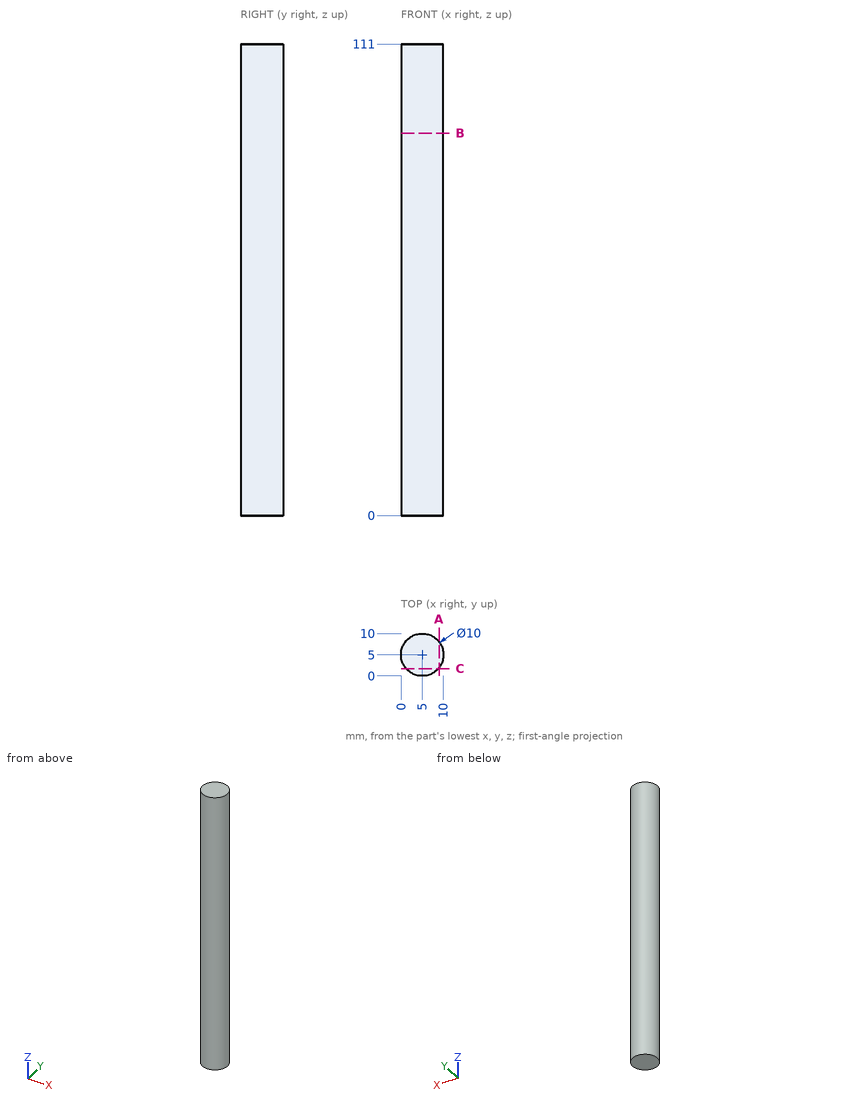
Print and shaded views of the part. All mm, measured from the part's lowest x, y and z. Round coordinates to 2 decimals unless told otherwise and drop trailing zeros. Write each loop counter-clockwise with the first axis right and the second up, starting at its lowest first coordinate (ties: lowest second). Pieces come first, ordered by that corner, then holes. Notation, with made-up numbers: (-16.5, 42) - (40.5, 42) arc R21 ccw to (40.5, 57) - close; hole circle Ø10 at (66, -32). An arc over 180 degrees is marked (long way). Use CSV: the item, a comma, the result in double quotes. Start each with the question number.
Item 1: Pin check, flat tips, straight feed: P1, Ø6, axis at x = 6.5, z = 33, coming from the +Y side; P2, Ø2, axis at y = 3, z = 33, coming from the -X side. Stop position of each tip, or through.
Item 2: Band-saw the part on B-B (z = 90). Write the cut outline in (x, y).
Item 3: Drill centre lines: L1, parallel to X at y = 4.75, z = 57; L2, parallel to X at y = 9, z = 88. Where is each one in solid material? Low to high. Write a range as [from, to].
Item 4: Band-saw the part on C-C (y = 1.75). Write the cut outline in (x, z).
Item 5: Band-saw the part on A-A (x = 9). Write the cut outline in (y, z).
Checked values:
1,P1,"stops at y = 10"
1,P2,"stops at x = 0.1"
2,outline,"circle Ø10 at (5, 5)"
3,L1,"x = [0.01, 9.99]"
3,L2,"x = [2, 8]"
4,outline,"(1.2, 0) - (8.8, 0) - (8.8, 111) - (1.2, 111) - close"
5,outline,"(2, 0) - (8, 0) - (8, 111) - (2, 111) - close"
